Here's how the part is built. I have some questions about the finished solid (model axes, mm). Face numbers are marked on the shaded views. A direction names the side the tool comes from. Give positions to 0.01 mm unless a question says otherwise; leave off trailing zeros. Loops run counter-clockwise (first coordinate to the right, second up) from the corner with the lowest first, then second, coordinate; pieces in that order, holes last.
Q1. Will these pins go through, and if not, where does the flat tip stop? P1, Ø2.5, axis at y = 1.5, z = 15, coming from the +X side; P2, Ø0.5, axis at x = 0, y = 1.5, coming from the +Z side; P3, Ø1, axis at x = 5, z = 22.5, coming from the +Y side; P4, Ø1.5, axis at x = -10.5, y = 8.5, coming from the +Z side.
Q2. If we section it at C-C (x = 0): Please give me the cut outline in (y, z) (3 decimals), plus the area to 3 significant figures.
Q3. If we section it at A-A (x = -9.5): Please give me the cut outline in (y, z).
Q4. If we section it at B-B (y = 8.5): Please give me the cut outline in (x, z) (1 decimal), plus the area to 3 significant figures.
Q5. For the marked faces 1, 2, 3, 4 and 5, which set-ups out of +Z, -Z, +X, -X, +Y, -Y let a thin tool reach every point of the face, with its end or its side?
Q6. We'd pull the mould along Z, two halves only. Please class the marked faces 6, 7 and 8: +Z half, -Z half, draft (parallel to the pull), parting line (faces both ways), or undercut.
Q7. If we section it at D-D (z = -20.5): Please give me the cut outline in (x, y).
Q8. I need wall thicknesses on line 1 (Z direction, x = -9, y = 1); line 2 (Z direction, x = 9, y = 2.25); line 3 (Y direction, x = -6, z = -2). Which ranges of each line are inside material? Lowest first, please.
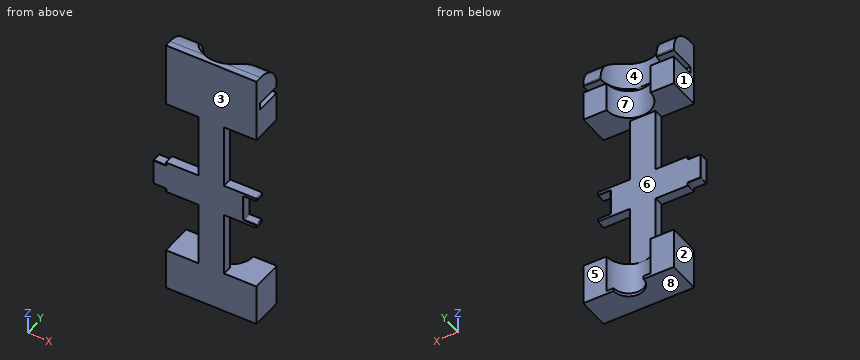
from build123d import *

# Parameters (mm, degrees)
SKETCH1_W                   = 28
SKETCH1_H                   = 90
BOSS_EXTRUDE1_DEPTH         = 10
SKETCH4_W                   = 6.8
SKETCH4_H                   = 71
SKETCH5_W                   = 28
SKETCH5_H                   = 2.2
FLANGE_SLOT_DEPTH           = 8.2
SKETCH6_W                   = 8.632931683
SKETCH6_H                   = 8.632931683
SKETCH3_W                   = 4.625
SKETCH3_H                   = 10.2
CUT_EXTRUDE4_DEPTH          = 49.176757882
CUT_EXTRUDE4_DEPTH_BACK     = 49.176757882
SKETCH17_W                  = 38.089842412
SKETCH17_H                  = 14.4
SKETCH18_W                  = 28
SKETCH18_H                  = 50
SYRINGE_BAY_DEPTH           = 7
SYRINGE_PLUNGER_LEFT_R      = 8
SYRINGE_START               = -15
SYRINGE_PLUNGER_RIGHT_DEPTH = 23.632931783
SKETCH19_W                  = 10
SKETCH19_H                  = 20
CUT_EXTRUDE5_DEPTH          = 10
SKETCH24_W                  = 8
SKETCH24_H                  = 3
BOSS_EXTRUDE3_DEPTH         = 4
SKETCH25_W                  = 8
SKETCH25_H                  = 3
CUT_EXTRUDE6_DEPTH          = 4
FILLET1_R                   = 0.2
FILLET2_R                   = 0.2


with BuildPart() as part:
    # Sketch1 → Boss-Extrude1 (new body)
    with BuildSketch(Plane(origin=(0, 0, 0), x_dir=(1, 0, 0), z_dir=(0, 1, 0))):
        Rectangle(SKETCH1_W, SKETCH1_H)
    extrude(amount=BOSS_EXTRUDE1_DEPTH)

    # Sketch4 → Syringe Body slot (revolve, cut)
    with BuildSketch(Plane(origin=(0, 10, 0), x_dir=(1, 0, 0), z_dir=(0, 1, 0))):
        with Locations((-3.4, 1.3)):
            Rectangle(SKETCH4_W, SKETCH4_H)
    revolve(axis=Axis((0, 10, -36.8), (0, 0, 1)), mode=Mode.SUBTRACT)

    # Sketch5 → Flange Slot (cut)
    with BuildSketch(Plane(origin=(0, 10, 0), x_dir=(1, 0, 0), z_dir=(0, 1, 0))):
        with Locations((0, -35.267068317)):
            Rectangle(SKETCH5_W, SKETCH5_H)
    extrude(amount=-FLANGE_SLOT_DEPTH, mode=Mode.SUBTRACT)

    # Sketch6 → Plunger Slot (revolve, cut)
    with BuildSketch(Plane(origin=(0, 10, 0), x_dir=(1, 0, 0), z_dir=(0, 1, 0))):
        with Locations((-4.316465842, -40.683534159)):
            Rectangle(SKETCH6_W, SKETCH6_H)
    revolve(axis=Axis((0, 10, 45), (0, 0, -1)), mode=Mode.SUBTRACT)

    # Sketch3 → Barrell Slot (revolve, cut)
    with BuildSketch(Plane(origin=(0, 10, 0), x_dir=(1, 0, 0), z_dir=(0, 1, 0))):
        with Locations((-2.3125, 39.9)):
            Rectangle(SKETCH3_W, SKETCH3_H)
    revolve(axis=Axis((0, 10, -45), (0, 0, 1)), mode=Mode.SUBTRACT)

    # Sketch17 → Cut-Extrude4 (cut, two sides: drawn at the far end of the back side and taken through both)
    with BuildSketch(Plane(origin=(0, 10, 0), x_dir=(1, 0, 0), z_dir=(0, 1, 0)).offset(-CUT_EXTRUDE4_DEPTH_BACK)):
        with Locations((0, 45)):
            Rectangle(SKETCH17_W, SKETCH17_H)
    extrude(amount=CUT_EXTRUDE4_DEPTH + CUT_EXTRUDE4_DEPTH_BACK, mode=Mode.SUBTRACT)

    # Sketch18 → Syringe Bay (cut)
    with BuildSketch(Plane(origin=(0, 10, 0), x_dir=(1, 0, 0), z_dir=(0, 1, 0))):
        Rectangle(SKETCH18_W, SKETCH18_H)
    extrude(amount=-SYRINGE_BAY_DEPTH, mode=Mode.SUBTRACT)

    # Syringe plunger left
    syringe_plunger_left_edges = [part.edges().sort_by_distance(p)[0] for p in [
        (11.316465842, 10, 45),
    ]]
    fillet(syringe_plunger_left_edges, radius=SYRINGE_PLUNGER_LEFT_R)

    # Syringe plunger right: read off the stored shape, not the designer's step
    # Syringe plunger right outline → Syringe plunger right (cut)
    with BuildSketch(Plane.YZ.offset(SYRINGE_START)):
        with BuildLine():
            ThreePointArc((2, 45), (7.656854249, 42.656854249), (10, 37))
            Line((10, 37), (10, 45))
            Line((10, 45), (2, 45))
        make_face()
    extrude(amount=SYRINGE_PLUNGER_RIGHT_DEPTH, mode=Mode.SUBTRACT)

    # Sketch19 → Cut-Extrude5 (cut)
    with BuildSketch(Plane(origin=(0, 3, 0), x_dir=(1, 0, 0), z_dir=(0, 1, 0))):
        with Locations((-9, 15)):
            Rectangle(SKETCH19_W, SKETCH19_H)
        with Locations((-9, -15)):
            Rectangle(SKETCH19_W, SKETCH19_H)
        with Locations((9, -15)):
            Rectangle(SKETCH19_W, SKETCH19_H)
        with Locations((9, 15)):
            Rectangle(SKETCH19_W, SKETCH19_H)
    extrude(amount=-CUT_EXTRUDE5_DEPTH, mode=Mode.SUBTRACT)

    # Sketch24 → Boss-Extrude3 (add)
    with BuildSketch(Plane.ZY.offset(14)):
        with Locations((0, 1.5)):
            Rectangle(SKETCH24_W, SKETCH24_H)
    extrude(amount=BOSS_EXTRUDE3_DEPTH)

    # Sketch25 → Cut-Extrude6 (cut)
    with BuildSketch(Plane(origin=(14, 0, 0), x_dir=(0, 0, -1), z_dir=(1, 0, 0))):
        with Locations((0, 1.5)):
            Rectangle(SKETCH25_W, SKETCH25_H)
    extrude(amount=-CUT_EXTRUDE6_DEPTH, mode=Mode.SUBTRACT)

    # Fillet1
    fillet1_edges = [part.edges().sort_by_distance(p)[0] for p in [
        (14, 0, 4.5),
        (14, 3, 4.5),
        (14, 1.5, -5),
        (14, 1.5, 5),
        (14, 0, -4.5),
        (14, 3, -4.5),
        (10, 1.5, -4),
        (12, 3, -4),
        (10, 0, 0),
        (12, 0, -4),
        (10, 1.5, 4),
        (12, 0, 4),
        (10, 3, 0),
        (12, 3, 4),
        (14, 1.5, -4),
        (14, 1.5, 4),
    ]]
    fillet(fillet1_edges, radius=FILLET1_R)

    # Fillet2
    fillet2_edges = [part.edges().sort_by_distance(p)[0] for p in [
        (-14, 0, -4.5),
        (-14, 3, -4.5),
        (-14, 3, 4.5),
        (-14, 0, 4.5),
        (-14, 1.5, 4),
        (-16, 0, 4),
        (-16, 3, 4),
        (-14, 1.5, -4),
        (-16, 3, -4),
        (-16, 0, -4),
        (-18, 1.5, 4),
        (-18, 3, 0),
        (-18, 1.5, -4),
        (-18, 0, 0),
    ]]
    fillet(fillet2_edges, radius=FILLET2_R)


solid = part.part
Check sheet entries:
1. P1: stops at x = 4
1. P2: stops at z = 45
1. P3: passes through
1. P4: stops at z = 42.56
2. outline: (0, -37.8) - (5.375, -37.8) - (5.375, -36.8) - (3.2, -36.8) - (3.2, -25) - (3, -25) - (3, 25) - (3.2, 25) - (3.2, 34.167) - (1.8, 34.167) - (1.8, 36.367) - (1.367, 36.367) - (1.367, 45) - (0, 45) - close
2. area: 238 mm2
3. outline: (0, -37.8) - (10, -37.8) - (10, -25) - (0, -25) - close; (0, -5) - (3, -5) - (3, 5) - (0, 5) - close; (0, 25) - (10, 25) - (10, 34.17) - (1.8, 34.17) - (1.8, 36.37) - (10, 36.37) - (10, 37) arc R8 ccw to (2, 45) - (0, 45) - close
4. outline: (-14, -37.8) - (-4.4, -37.8) - (-4.4, -36.8) - (-6.6, -36.8) - (-6.6, -25) - (-14, -25) - close; (-14, 25) - (-6.6, 25) - (-6.6, 34.2) - (-14, 34.2) - close; (-14, 36.4) - (-8.5, 36.4) - (-8.5, 41.7) - (-14, 41.7) - close; (4.4, -37.8) - (14, -37.8) - (14, -25) - (6.6, -25) - (6.6, -36.8) - (4.4, -36.8) - close; (6.6, 25) - (14, 25) - (14, 34.2) - (6.6, 34.2) - close; (8.5, 36.4) - (14, 36.4) - (14, 41.7) - (8.5, 41.7) - close
4. area: 386 mm2
5. face 1: +Z, -X, +Y, -Y
5. face 2: -Z, -X, +Y, -Y
5. face 3: +Z, -Z, +X, -X, -Y
5. face 4: +Z, +Y
5. face 5: +Z, -Z, +X, -X, +Y
6. face 6: undercut
6. face 7: draft
6. face 8: -Z half
7. outline: (-4, 0) - (4, 0) - (4, 3) - (-4, 3) - close
8. line 1: z = -37.8 to -25, -5 to 5, 25 to 45
8. line 2: z = -37.8 to -25, -5 to 5, 25 to 34.17, 36.37 to 45
8. line 3: y = 0 to 3
